Model file for the job. Use its own axes, mm. Face numbers are marked on the shaded views. A direction names the side the tool comes from. Round coordinates to 2 decimals unless told otherwise and drop trailing zeros. Order: outer loops, then holes, each group sorted by start corner. A loop starts at its lowest first (then second) coordinate and runs counter-clockwise, first axis right, second up. Notation, with made-up numbers: (7, 14.25) -> (23, 14.25) arc R16 cw to (23, 45.25) -> close; hole circle Ø5 at (10, 57.25). An arc over 180 degrees is marked (long way). Answer as CSV lines item,"result".
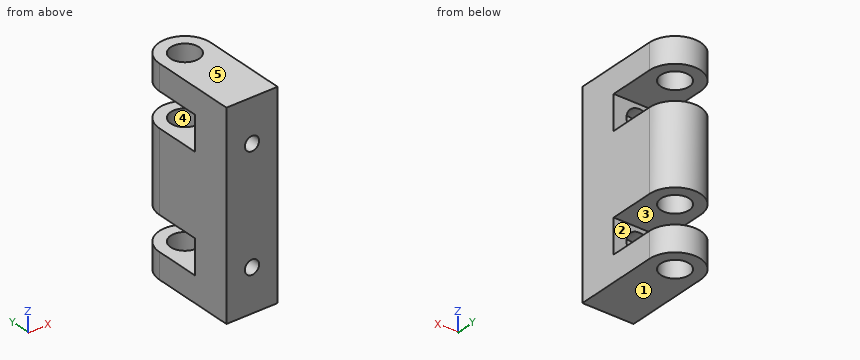
Autodesk Inventor part; units mm, degrees
ref_plane "YZ Plane" through (0, 0, 0) normal (1, 0, 0) x (0, 1, 0)
ref_plane "XZ Plane" through (0, 0, 0) normal (0, 1, 0) x (-1, 0, 0)
ref_plane "XY Plane" through (0, 0, 0) normal (0, 0, 1) x (1, 0, 0)
sketch "Esboço1" plane through (0, 0, 0) normal (0, 0, 1) x (1, 0, 0)
  arc A0 (9, 0) -> (-9, 0) centre (0, 0) ccw
  line L0 (-9, 0) -> (-9, -30)
  line L1 (-9, -30) -> (9, -30)
  line L2 (9, -30) -> (9, 0)
  dimension "d1" = 9
  dimension "d2" = 30
extrude "Extrusão1" add sketch "Esboço1" along normal mid plane 70
sketch "Esboço2" plane through (0, 0, 0) normal (1, 0, 0) x (0, 1, 0)
  line L0 (9, -35) -> (9, 35)
  line L1 (9, 26) -> (-16, 26)
  line L2 (-16, 26) -> (-16, 14)
  line L3 (-16, 14) -> (9, 14)
  line L4 (9, 14) -> (9, 26)
  line L5 (9, -14) -> (-16, -14)
  line L6 (-16, -14) -> (-16, -26)
  line L7 (-16, -26) -> (9, -26)
  line L8 (9, -26) -> (9, -14)
  line L9 (-30, -35) -> (-30, 35)
  point P0 (0, 0)
  point P1 (-16, -20)
  point P2 (-16, 20)
  dimension "d5" = 12
  dimension "d6" = 14
  dimension "d7" = 14
  dimension "d8" = 14
  dimension "d9" = 12
extrude "Extrusão2" cut sketch "Esboço2" along normal mid plane 20
sketch "Esboço3" plane through (0, 0, 35) normal (0, 0, 1) x (1, 0, 0)
  circle A0 centre (0, 0) radius 5
  dimension "d12" = 10
extrude "Extrusão3" cut sketch "Esboço3" against normal through all
sketch "Esboço4" plane through (-9, -16, 26) normal (0, 1, 0) x (1, 0, 0)
  point P0 (9, 26)
  point P1 (9, 6)
  point P2 (9, 46)
  dimension "d15" = 20
  dimension "d16" = 20
hole "Furo1" at (0, -16, 20) at (0, -16, -20) direction (0, -1, 0) diameter 5 end through all counterbore diameter 9 counterbore depth 5
Q1. Mould opens along Z. For the marked faces 3, 4 and 5 say: +Z half, -Z half, draft (parallel to the pull), parting line (faces both ways), or undercut.
Checks:
face 3,"undercut"
face 4,"draft"
face 5,"+Z half"
Q2. Saw through at A-A (z = 20). Write the cut outline in (x, y), plus the area to 3 significant figures.
Checks:
outline,"(-9, -30) -> (-2.5, -30) -> (-2.5, -21) -> (-4.5, -21) -> (-4.5, -16) -> (-9, -16) -> close; (2.5, -30) -> (9, -30) -> (9, -16) -> (4.5, -16) -> (4.5, -21) -> (2.5, -21) -> close"
area,"162 mm²"
Q3. Flat gauge pins, fed straight in: pin 1 (10 mm diameter, centred on x = -0.5, z = 19.5, fed in from +Y); pin 2 (8 mm diameter, centred on x = 0, z = 20, fed in from +Y). Where does each tip first touch, or does it go through?
Checks:
pin 1,"y = -16"
pin 2,"y = -21"
Q4. Saw through at B-B (y = -10). Write the cut outline in (x, z).
Checks:
outline,"(-9, -35) -> (9, -35) -> (9, -26) -> (-9, -26) -> close; (-9, -14) -> (9, -14) -> (9, 14) -> (-9, 14) -> close; (-9, 26) -> (9, 26) -> (9, 35) -> (-9, 35) -> close"
Q5. Wall check: L1, parallel to Z at x = -8.25, y = 0; L2, parallel to X at y = -19.5, z = -20; L3, parallel to Y at x = 1, z = -24. Give the ranges that are in metal, low to high. Write a range as [from, to].
Checks:
L1,"[-35, -26], [-14, 14], [26, 35]"
L2,"[-9, -4.5], [4.5, 9]"
L3,"[-30, -21]"
Q6. Saw through at D-D (x = 0). State how many separate pieces and enclosed holes the cut face has, plus the area to 3 significant figures.
Checks:
separate pieces,"6"
enclosed holes,"0"
area,"1,490 mm²"
Q7. Tool access for the marked faces 1 and 2: list every direction of +Z, -Z, +X, -X, +Y, -Y with a clear straight run to the whole face (end or side of a thin tool).
Checks:
face 1,"-Z, +X, -X, +Y, -Y"
face 2,"+X, -X, +Y"
Q8. Saw through at C-C (z = 9.5). Write the cut outline in (x, y), plus the area to 3 significant figures.
Checks:
outline,"(-9, -30) -> (9, -30) -> (9, 0) arc R9 ccw to (-9, 0) -> close; hole circle Ø10 at (0, 0)"
area,"589 mm²"
